Check sheet for the modelled part. Datum: model origin and axes. Units: mm. A direction names the side the tool comes from. Coordinates: 2 decimals unless noted, no trailing zeros. Loops run counter-clockwise (first coordinate to the right, second up) from the corner with the lowest first, then second, coordinate; pieces in that order, holes last. Notation, with made-up numbers: (-21.5, 59) -> (37.5, 59) arc R9 cw to (37.5, 65) -> close; hole circle Ø11 at (12.5, 46). An arc over 180 degrees is marked (long way). Use one line per item in the form item = value.
from build123d import *

# Parameters (mm, degrees)
SKETCH1_W           = 80.1
SKETCH1_H           = 42
SKETCH1_R           = 1.25
BOSS_EXTRUDE1_DEPTH = 2.6
SKETCH2_W           = 80.1
SKETCH2_H           = 42
SKETCH2_W_2         = 76.1
SKETCH2_H_2         = 37.9
BOSS_EXTRUDE2_DEPTH = 1
FILLET1_R           = 2
FILLET2_R           = 1.5
SKETCH3_W           = 13
SKETCH3_H           = 5.85
CUT_EXTRUDE1_DEPTH  = 49.913903954
SKETCH4_W           = 7.8
SKETCH4_H           = 1.2
CUT_EXTRUDE2_DEPTH  = 49.913903954
SKETCH5_W           = 6.8
SKETCH5_H           = 1.8
CUT_USB_DEPTH       = 4
SKETCH6_W           = 11.2
SKETCH6_H           = 3.25
CUT_PILL_DEPTH      = 2.6


with BuildPart() as part:
    # Sketch1 → Boss-Extrude1 (new body)
    with BuildSketch(Plane.XY):
        with Locations((4.05, 0)):
            Rectangle(SKETCH1_W, SKETCH1_H)
        with Locations((39.55, -16.4)):
            Circle(SKETCH1_R, mode=Mode.SUBTRACT)
        with Locations(Location((-31.45, -16.4, 0), (0, 0, 180))):
            Circle(SKETCH1_R, mode=Mode.SUBTRACT)
        with Locations(Location((39.55, 16.4, 0), (0, 0, 180))):
            Circle(SKETCH1_R, mode=Mode.SUBTRACT)
        with Locations((-31.45, 16.4)):
            Circle(SKETCH1_R, mode=Mode.SUBTRACT)
        with BuildLine():
            Line((35.916819575, -17.75), (-27.816819575, -17.75))
            ThreePointArc((-27.816819575, -17.75), (-28.557052785, -17.422350202), (-28.812211472, -16.654109589))
            ThreePointArc((-28.812211472, -16.654109589), (-29.57616703, -14.52616703), (-31.704109589, -13.762211472))
            ThreePointArc((-31.704109589, -13.762211472), (-32.472350202, -13.507052785), (-32.8, -12.766819575))
            Line((-32.8, -12.766819575), (-32.8, 14.5))
            Line((-32.8, 14.5), (-28.8, 14.5))
            Line((-28.8, 14.5), (-28.8, 17.75))
            Line((-28.8, 17.75), (-27.816819575, 17.75))
            Line((-27.816819575, 17.75), (35.916819575, 17.75))
            ThreePointArc((35.916819575, 17.75), (36.657052785, 17.422350202), (36.912211472, 16.654109589))
            ThreePointArc((36.912211472, 16.654109589), (37.67616703, 14.52616703), (39.804109589, 13.762211472))
            ThreePointArc((39.804109589, 13.762211472), (40.572350202, 13.507052785), (40.9, 12.766819575))
            Line((40.9, 12.766819575), (40.9, -12.766819575))
            ThreePointArc((40.9, -12.766819575), (40.572350202, -13.507052785), (39.804109589, -13.762211472))
            ThreePointArc((39.804109589, -13.762211472), (37.67616703, -14.52616703), (36.912211472, -16.654109589))
            ThreePointArc((36.912211472, -16.654109589), (36.657052785, -17.422350202), (35.916819575, -17.75))
        make_face(mode=Mode.SUBTRACT)
    extrude(amount=BOSS_EXTRUDE1_DEPTH)

    # Sketch2 → Boss-Extrude2 (add)
    with BuildSketch(Plane.XY.offset(2.6)):
        with Locations((4.05, 0)):
            Rectangle(SKETCH2_W, SKETCH2_H)
        with Locations((4.05, 0)):
            Rectangle(SKETCH2_W_2, SKETCH2_H_2, mode=Mode.SUBTRACT)
    extrude(amount=BOSS_EXTRUDE2_DEPTH)

    # Fillet1
    fillet1_edges = [part.edges().sort_by_distance(p)[0] for p in [
        (44.1, -21, 1.8),
        (-36, -21, 1.8),
        (-36, 21, 1.8),
        (44.1, 21, 1.8),
    ]]
    fillet(fillet1_edges, radius=FILLET1_R)

    # Fillet2
    fillet2_edges = [part.edges().sort_by_distance(p)[0] for p in [
        (-34, -18.95, 3.1),
        (42.1, -18.95, 3.1),
        (42.1, 18.95, 3.1),
        (-34, 18.95, 3.1),
    ]]
    fillet(fillet2_edges, radius=FILLET2_R)

    # Sketch3 → Cut-Extrude1 (cut, through all)
    with BuildSketch(Plane.XY.offset(2.6)):
        with Locations((-15, 16.025)):
            Rectangle(SKETCH3_W, SKETCH3_H)
    extrude(amount=-CUT_EXTRUDE1_DEPTH, mode=Mode.SUBTRACT)

    # Sketch4 → Cut-Extrude2 (cut, through all)
    with BuildSketch(Plane.XY.offset(2.6)):
        with Locations((-22.65, -18.35)):
            Rectangle(SKETCH4_W, SKETCH4_H)
    extrude(amount=-CUT_EXTRUDE2_DEPTH, mode=Mode.SUBTRACT)

    # Sketch5 → Cut-USB (cut)
    with BuildSketch(Plane.XZ.offset(21)):
        with Locations((-22.65, 1.7)):
            Rectangle(SKETCH5_W, SKETCH5_H)
    extrude(amount=-CUT_USB_DEPTH, mode=Mode.SUBTRACT)

    # Sketch6 → Cut-Pill (cut)
    with BuildSketch(Plane(origin=(0, 0, 0), x_dir=(-1, 0, 0), z_dir=(0, 0, -1))):
        with Locations((1.8, 19.375)):
            Rectangle(SKETCH6_W, SKETCH6_H)
    extrude(amount=-CUT_PILL_DEPTH, mode=Mode.SUBTRACT)


solid = part.part
(1) Mould release check, pull along X, two halves, no side actions. Record for faces 1 (the flat face through (1, -20, 3.6)), 2 (the flat face through (-23, -20, 2.6)), 3 (the cylindrical face through (-35.43, 20.4, 1.77)): +X half, -X half, draft (parallel to the pull), parting line (faces both ways), or undercut.
Established:
face_1 = draft
face_2 = undercut
face_3 = -X half
(2) Section check B-B, the plane y = 10.5. Record the boundary of the cut face in (x, z), plus the area to 3 significant figures.
Established:
outline = (-36, 0) -> (-32.8, 0) -> (-32.8, 2.6) -> (-34, 2.6) -> (-34, 3.6) -> (-36, 3.6) -> close; (40.9, 0) -> (44.1, 0) -> (44.1, 3.6) -> (42.1, 3.6) -> (42.1, 2.6) -> (40.9, 2.6) -> close
area = 20.6 mm²
(3) Scan lines: line 1 along Y through (x, z) = (39.55, 1.35); line 2 along X through (y, z) = (13, 3.3); line 3 along Y through (x, z) = (15.5, 3). Record each from-to range of solid material in increasing order.
Established:
line_1 = -21 to -17.65, -15.15 to -13.75, 13.75 to 15.15, 17.65 to 21
line_2 = -36 to -34, 42.1 to 44.1
line_3 = -21 to -18.95, 18.95 to 21
(4) Section check D-D, the plane z = 1.45. Give the number of separate pieces and of enclosed holes in the cut face, plus the area to 3 significant figures.
Established:
separate_pieces = 2
enclosed_holes = 4
area = 707 mm²
(5) Tool access check on faces 4 (the cylindrical face through (-33.55, 18.52, 3.11)), 5 (the flat face through (-7.4, 19, 1)), 6 (the cylindrical face through (37.7, -14.5, 1.3)). Record the directions out of +Z, -Z, +X, -X, +Y, -Y that give a thin tool (end or side, any length) a straight path to the whole face; none if there is none.
Established:
face_4 = +Z
face_5 = -Z, +Y
face_6 = +Z, -Z
(6) Section check C-C, the plane x = 24.5. Record the boundary of the cut face in (y, z), plus the area to 3 significant figures.
Established:
outline = (-21, 0) -> (-17.75, 0) -> (-17.75, 2.6) -> (-18.95, 2.6) -> (-18.95, 3.6) -> (-21, 3.6) -> close; (17.75, 0) -> (21, 0) -> (21, 3.6) -> (18.95, 3.6) -> (18.95, 2.6) -> (17.75, 2.6) -> close
area = 21.0 mm²
(7) Go/stop test with flat-tipped pins: P1, Ø3, axis at x = 39.55, y = 16.4, coming from the +Z side; P2, Ø1, axis at x = -0.5, y = 20, coming from the -Z side. Record where each tip stops, or that it passes through.
Established:
P1 = 2.6
P2 = 2.6
(8) Section check A-A, the plane x = -11.5. Record the boundary of the cut face in (y, z).
Established:
outline = (-21, 0) -> (-17.75, 0) -> (-17.75, 2.6) -> (-18.95, 2.6) -> (-18.95, 3.6) -> (-21, 3.6) -> close; (18.95, 0) -> (21, 0) -> (21, 3.6) -> (18.95, 3.6) -> close
